Model file for the job. Use its own axes, mm. Face numbers are marked on the shaded views. A direction names the side the tool comes from. Round coordinates to 2 decimals unless told otherwise and drop trailing zeros. Order: outer loops, then holes, each group sorted by start corner. A loop starts at its lowest first (then second) coordinate and runs counter-clockwise, first axis right, second up. Notation, with made-up numbers: (-40, 23.25) - (4, 23.25) arc R33 ccw to (4, 58.25) - close; hole circle Ø4 at (65.5, -0.5). An arc over 180 degrees is marked (long way). Use one line per item in the form item = value.
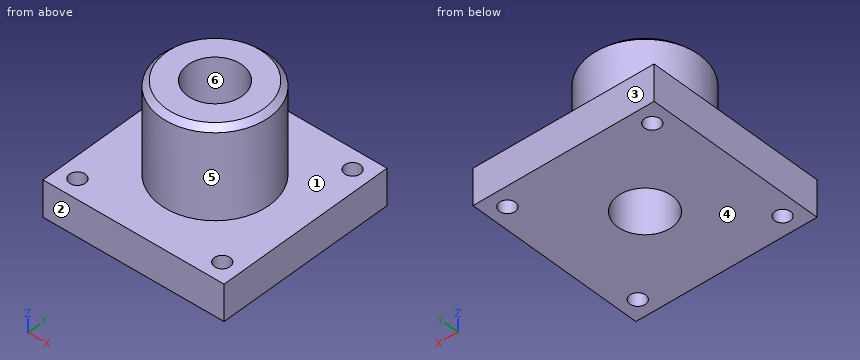
from build123d import *

# Parameters (mm, degrees)
SKETCH1_W                    = 254
SKETCH1_H                    = 254
BOSS_EXTRUDE1_DEPTH          = 50.8
SKETCH2_R                    = 76.2
BOSS_EXTRUDE2_DEPTH          = 127
CHAMFER1_SIZE                = 7.62
SKETCH3_R                    = 38.1
CUT_EXTRUDE1_DEPTH           = 178.8
F_7_8_0_875_DIAMETER_HOLE1_D = 22.225


with BuildPart() as part:
    # Sketch1 → Boss-Extrude1 (new body)
    with BuildSketch(Plane.XY):
        Rectangle(SKETCH1_W, SKETCH1_H)
    extrude(amount=BOSS_EXTRUDE1_DEPTH)

    # Sketch2 → Boss-Extrude2 (add)
    with BuildSketch(Plane.XY.offset(50.8)):
        Circle(SKETCH2_R)
    extrude(amount=BOSS_EXTRUDE2_DEPTH)

    # Chamfer1
    chamfer1_edges = [part.edges().sort_by_distance(p)[0] for p in [
        (-76.2, 0, 177.8),
    ]]
    chamfer(chamfer1_edges, length=CHAMFER1_SIZE)

    # Sketch3 → Cut-Extrude1 (cut, through all)
    with BuildSketch(Plane.XY.offset(177.8)):
        Circle(SKETCH3_R)
    extrude(amount=-CUT_EXTRUDE1_DEPTH, mode=Mode.SUBTRACT)

    # 7/8 (0.875) Diameter Hole1 (through all)
    with Locations(Plane.XY.offset(50.8)):
        with Locations((-101.6, 101.6), (101.6, 101.6), (101.6, -101.6), (-101.6, -101.6)):
            Hole(F_7_8_0_875_DIAMETER_HOLE1_D / 2)


solid = part.part
(1) Pin check, flat tip, straight feed: pin 1 (20 mm diameter, centred on x = -101.6, y = 101.6, fed in from +Z). Stop position of the tip, or through.
Report:
pin_1 = through
(2) Slice it at D-D on y = -101.6. Give the cut face in (x, z), then the cut area to 3 significant figures.
Report:
outline = (-127, 0) - (-112.71, 0) - (-112.71, 50.8) - (-127, 50.8) - close; (-90.49, 0) - (90.49, 0) - (90.49, 50.8) - (-90.49, 50.8) - close; (112.71, 0) - (127, 0) - (127, 50.8) - (112.71, 50.8) - close
area = 10,600 mm2
(3) Slice it at A-A on y = 0. Give the cut face in (x, z).
Report:
outline = (-127, 0) - (-38.1, 0) - (-38.1, 177.8) - (-68.58, 177.8) - (-76.2, 170.18) - (-76.2, 50.8) - (-127, 50.8) - close; (38.1, 0) - (127, 0) - (127, 50.8) - (76.2, 50.8) - (76.2, 170.18) - (68.58, 177.8) - (38.1, 177.8) - close
(4) Tool access for the marked faces 1 and 2: list every direction of +Z, -Z, +X, -X, +Y, -Y with a clear straight run to the whole face (end or side of a thin tool).
Report:
face_1 = +Z
face_2 = +Z, -Z, +X, -X, -Y
(5) Pull direction Y, two halves, no side cores. Call the marked faces 3, 4, 5 and 6: released by +Y, released by -Y, zero draft, split by the parting line, or undercut.
Report:
face_3 = released by +Y
face_4 = zero draft
face_5 = split by the parting line
face_6 = undercut
(6) Slice it at C-C on z = 42. Give the cut face in (x, y) (1 decimal).
Report:
outline = (-127, -127) - (127, -127) - (127, 127) - (-127, 127) - close; hole circle Ø22.2 at (-101.6, -101.6); hole circle Ø22.2 at (-101.6, 101.6); hole circle Ø76.2 at (0, 0); hole circle Ø22.2 at (101.6, -101.6); hole circle Ø22.2 at (101.6, 101.6)
(7) Probe probe 1 along Y at (x, z) = (-101.6, 20); probe 2 along X at (y, z) = (101, 30); probe 3 along Z at (x, y) = (110, -16.5). List the from-to ranges inside material, lowest first. Write a range as [from, to].
Report:
probe_1 = [-127, -112.71], [-90.49, 90.49], [112.71, 127]
probe_2 = [-127, -112.7], [-90.5, 90.5], [112.7, 127]
probe_3 = [0, 50.8]
